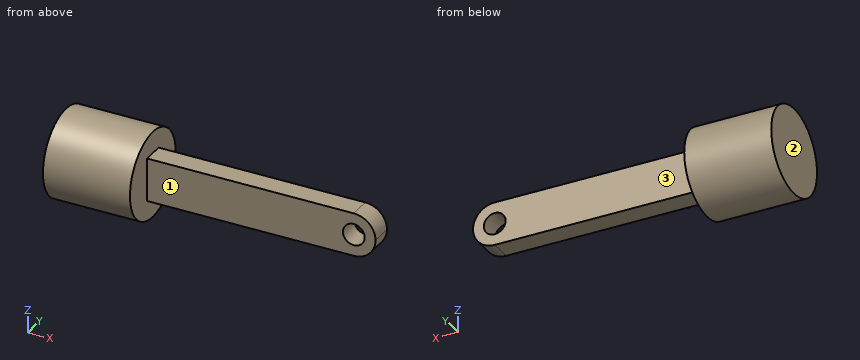
from build123d import *

# Parameters (mm, degrees)
F0_R     = 25.4
F1_DEPTH = 50.8
F2_W     = 12.7
F2_H     = 25.4
F3_DEPTH = 133.35
F4_R     = 12.69999
F5_R     = 6.35
F6_DEPTH = 31.751


# Not quite as in the source:
# - a fillet or chamfer is up to 0.001 mm smaller than in the source, because OpenCascade refuses the exact size


with BuildPart() as f1:
    # F0 (on Right) → F1 (new body)
    with BuildSketch(Plane.YZ):
        Circle(F0_R)
    extrude(amount=-F1_DEPTH)

    # F2 (on face) → F3 (join)
    with BuildSketch(Plane.YZ):
        Rectangle(F2_W, F2_H)
    extrude(amount=F3_DEPTH)

    # F4 (radius 12.7 in the source; OpenCascade refuses exactly that, so slightly less here)
    f4_edges = [f1.edges().sort_by_distance(p)[0] for p in [
        (133.35, 0, 12.7),
        (133.35, 0, -12.7),
    ]]
    fillet(f4_edges, radius=F4_R)

    # F5 (on face) → F6 (cut, through all)
    with BuildSketch(Plane.XZ.offset(6.35)):
        with Locations((120.65, 0)):
            Circle(F5_R)
    extrude(amount=-F6_DEPTH, mode=Mode.SUBTRACT)


solid = f1.part
Source: CAD feature listing. Evaluate the final solid. Frame: model axes, mm. Face numbers are marked on the shaded views. A direction names the side the tool comes from. Give positions to 0.01 mm unless a question says otherwise; leave off trailing zeros. Order: outer loops, then holes, each group sorted by start corner. A loop starts at its lowest first (then second) coordinate and runs counter-clockwise, first axis right, second up. Notation, with made-up numbers: (38.5, 32.5) -> (61.5, 32.5) arc R28 cw to (61.5, 55.5) -> close; hole circle Ø2 at (23.5, 6). An arc over 180 degrees is marked (long way). Use a Markdown table: item, result.
1) Reachability of the marked faces 1, 2 and 3 from +Z, -Z, +X, -X, +Y, -Y: full face, straight path, thin tool, end or side. Return the list, or none.
Answer list:
| item | result |
|---|---|
| face 1 | +Z, -Z, +X, -Y |
| face 2 | +Z, -Z, -X, +Y, -Y |
| face 3 | +Z, -Z, +X, +Y |
2) Section query D-D, the plane y = -19. Return the cut outline in (x, z), then the cut area to 3 significant figures.
Answer list:
| item | result |
|---|---|
| outline | (-50.8, -16.86) -> (0, -16.86) -> (0, 16.86) -> (-50.8, 16.86) -> close |
| area | 1,710 mm² |
3) Contact query for flat-ended pins moving along their axis: P1, Ø20.5, axis at x = 120.65, z = 0, coming from the -Y side; P2, Ø1, axis at x = 46.5, z = 3, coming from the +Y side; P3, Ø1.5, axis at x = 64.5, y = 6, coming from the +Z side. Output: stop coordinate, or through.
Answer list:
| item | result |
|---|---|
| P1 | y = -6.35 |
| P2 | y = 6.35 |
| P3 | z = 12.7 |
4) Ray query, line 1 along Y through (x, z) = (12.5, -7); line 2 along X through (y, z) = (22, -12); line 3 along Z through (x, y) = (51.5, 2). Return the intervals inside material, ascending. Write a range as [from, to].
Answer list:
| item | result |
|---|---|
| line 1 | [-6.35, 6.35] |
| line 2 | [-50.8, 0] |
| line 3 | [-12.7, 12.7] |
5) Section query C-C, the plane x = -28. Return the cut outline in (y, z).
Answer list:
| item | result |
|---|---|
| outline | circle Ø50.8 at (0, 0) |
6) Section query B-B, the plane z = -8.5. Return the cut outline in (x, y).
Answer list:
| item | result |
|---|---|
| outline | (-50.8, -23.94) -> (0, -23.94) -> (0, -6.35) -> (130.09, -6.35) -> (130.09, 6.35) -> (0, 6.35) -> (0, 23.94) -> (-50.8, 23.94) -> close |
